from build123d import *

# Parameters (mm, degrees)
F0_W        = 0.9483136237
F0_H        = 3.3681727946
F0_W_2      = 28.0582979321
F0_H_2      = 55.2397826687
F0_W_3      = 6.7223012447
F0_H_3      = 9.4989053905
F0_H_4      = 10.2295875549
F0_W_4      = 6.8684406579
F0_W_5      = 7.014580071
F0_H_5      = 9.6450410783
F0_H_6      = 9.9373161793
F0_W_6      = 10.7689313591
F0_H_7      = 1.450072974
F0_W_7      = 10.0600272417
F1_DEPTH    = 2.54
F2_R        = 0.889
F3_DEPTH    = 1.778
F4_T4_DEPTH = 15.6041495789
F4_T9_DEPTH = 15.6041495789
F5_DEPTH    = 3.81
F6_DEPTH    = 3.302


# Not quite as in the source:
# - a fillet or chamfer that OpenCascade refuses, or shapes differently, is made with other operations: its cross-section is extruded or revolved along the edge and cut away or added


with BuildPart() as f1:
    # F0 (on Top) → F1 (new body)
    with BuildSketch(Plane.XY):
        with Locations((-55.3537514061, 60.8582701534)):
            Rectangle(F0_W, F0_H)
        Polygon((-69.7804093361, 57.7241107821), (-69.7804093361, 55.3859174252), (-41.8754070997, 55.3859174252), (-41.8754070997, 57.7241107821), (-44.8195673525, 57.7241107821), (-54.8795945942, 57.7241107821), (-55.8279082179, 57.7241107821), (-56.7762218416, 57.7241107821), (-67.5451532006, 57.7241107821), align=None)
        Polygon((-75.3612667322, 53.0477277935), (-69.7804093361, 53.0477277935), (-41.7221114039, 53.0477277935), (-35.9445475042, 53.0477277935), (-35.9445475042, 55.3859174252), (-41.8754070997, 55.3859174252), (-69.7804093361, 55.3859174252), (-75.3612667322, 55.3859174252), align=None)
        with Locations((-56.3020650297, 60.8582701534)):
            Rectangle(F0_W, F0_H)
        with Locations((-55.75126037, 25.4278364591)):
            Rectangle(F0_W_2, F0_H_2)
        with Locations((-62.9119724035, 14.8329045624)):
            Rectangle(F0_W_3, F0_H_3, mode=Mode.SUBTRACT)
        with Locations((-62.9119724035, 29.2273983359)):
            Rectangle(F0_W_3, F0_H_4, mode=Mode.SUBTRACT)
        with Locations((-48.2252072543, 14.8329045624)):
            Rectangle(F0_W_4, F0_H_3, mode=Mode.SUBTRACT)
        with Locations((-48.2252072543, 29.2273983359)):
            Rectangle(F0_W_4, F0_H_4, mode=Mode.SUBTRACT)
        with Locations((-63.0581118166, 44.571781531)):
            Rectangle(F0_W_5, F0_H_5, mode=Mode.SUBTRACT)
        with Locations((-48.2252072543, 44.4256439805)):
            Rectangle(F0_W_4, F0_H_6, mode=Mode.SUBTRACT)
        with Locations((-62.1606875211, 58.4491472691)):
            Rectangle(F0_W_6, F0_H_7)
        with Locations((-55.3537514061, 58.4491472691)):
            Rectangle(F0_W, F0_H_7)
        with Locations((-49.8495809734, 58.4491472691)):
            Rectangle(F0_W_7, F0_H_7)
        with Locations((-56.3020650297, 58.4491472691)):
            Rectangle(F0_W, F0_H_7)
    extrude(amount=F1_DEPTH)

    # F2
    f2_edges = [f1.edges().sort_by_distance(p)[0] for p in [
        (-54.879595, 60.85827, 2.54),
        (-56.776222, 60.85827, 2.54),
        (-55.827908, 62.542357, 2.54),
        (-56.776222, 62.542357, 1.27),
        (-54.879595, 62.542357, 1.27),
    ]]
    fillet(f2_edges, radius=F2_R)

    # F0 (on Top) → F3 (join)
    with BuildSketch(Plane.XY):
        with Locations((-63.0581118166, 44.571781531)):
            Rectangle(F0_W_5, F0_H_5)
        with Locations((-48.2252072543, 44.4256439805)):
            Rectangle(F0_W_4, F0_H_6)
        with Locations((-62.9119724035, 29.2273983359)):
            Rectangle(F0_W_3, F0_H_4)
        with Locations((-48.2252072543, 29.2273983359)):
            Rectangle(F0_W_4, F0_H_4)
        with Locations((-48.2252072543, 14.8329045624)):
            Rectangle(F0_W_4, F0_H_3)
        with Locations((-62.9119724035, 14.8329045624)):
            Rectangle(F0_W_3, F0_H_3)
    extrude(amount=F3_DEPTH)

    # F4: chamfer of 2.54 on 2 edges, made by hand


with BuildPart() as f4_tool2:
    # F4_s3 → F4_t4 (new body)
    with BuildSketch(Plane.XY.offset(-6.5320747894)):
        Polygon((-67.5451532006, 56.6341837561), (-65.0051532006, 59.1741837561), (-67.5451532006, 59.1741837561), align=None)
    extrude(amount=F4_T4_DEPTH)

    split(bisect_by=Plane.XZ.offset(-57.7241107821), keep=Keep.BOTTOM)


with BuildPart() as f1_1:
    add(f1.part)

    # F4_t1: cut F4_tool2
    add(f4_tool2.part, mode=Mode.SUBTRACT)


with BuildPart() as f4_tool7:
    # F4_s8 → F4_t9 (new body)
    with BuildSketch(Plane.XY.offset(-6.5320747894)):
        Polygon((-44.8195673525, 56.6341837561), (-47.3595673525, 59.1741837561), (-44.8195673525, 59.1741837561), align=None)
    extrude(amount=F4_T9_DEPTH)

    split(bisect_by=Plane.XZ.offset(-57.7241107821), keep=Keep.BOTTOM)


with BuildPart() as f1_2:
    add(f1_1.part)

    # F4_t6: cut F4_tool7
    add(f4_tool7.part, mode=Mode.SUBTRACT)

    # F0 (on Top) → F5 (join)
    with BuildSketch(Plane.XY):
        Polygon((-75.3612667322, 53.0477277935), (-69.7804093361, 53.0477277935), (-41.7221114039, 53.0477277935), (-35.9445475042, 53.0477277935), (-35.9445475042, 55.3859174252), (-41.8754070997, 55.3859174252), (-69.7804093361, 55.3859174252), (-75.3612667322, 55.3859174252), align=None)
    extrude(amount=F5_DEPTH)

    # F0 (on Top) → F6 (join)
    with BuildSketch(Plane.XY):
        Polygon((-69.7804093361, 57.7241107821), (-69.7804093361, 55.3859174252), (-41.8754070997, 55.3859174252), (-41.8754070997, 57.7241107821), (-44.8195673525, 57.7241107821), (-54.8795945942, 57.7241107821), (-55.8279082179, 57.7241107821), (-56.7762218416, 57.7241107821), (-67.5451532006, 57.7241107821), align=None)
    extrude(amount=F6_DEPTH)


solid = f1_2.part
Build history of the part. All positions in model axes, mm. A direction names the side the tool comes from. Round coordinates to 2 decimals unless told otherwise and drop trailing zeros. Write each loop counter-clockwise with the first axis right and the second up, starting at its lowest first coordinate (ties: lowest second). Pieces come first, ordered by that corner, then holes. Notation, with made-up numbers: (69.25, 36) -> (118.25, 36) arc R25 cw to (118.25, 52) -> close; hole circle Ø4 at (-35, 37). An arc over 180 degrees is marked (long way). Write item = value, one per line.
(1) Band-saw the part on B-B (y = 40.5). Give the cut face in (x, z), then the cut area to 3 significant figures.
Answer:
outline = (-69.78, 0) -> (-41.72, 0) -> (-41.72, 2.54) -> (-44.79, 2.54) -> (-44.79, 1.78) -> (-51.66, 1.78) -> (-51.66, 2.54) -> (-59.55, 2.54) -> (-59.55, 1.78) -> (-66.57, 1.78) -> (-66.57, 2.54) -> (-69.78, 2.54) -> close
area = 60.7 mm2
(2) Two-plate mould, pull along Y, no slides. Class faces 4 (the face through (-56, -2.192, 1)), 5 (the face through (-63, 45, 1.778)), 6 (the face through (-41.875, 57, 2)): pulls with the +Y half, pulls with the -Y half, needs draft (parallel to the pull), parting line crosses it, or undercut.
Answer:
face_4 = pulls with the -Y half
face_5 = undercut
face_6 = needs draft
(3) Band-saw the part on D-D (y = 31.5). Give the cut face in (x, z), then the cut area to 3 significant figures.
Answer:
outline = (-69.78, 0) -> (-41.72, 0) -> (-41.72, 2.54) -> (-44.79, 2.54) -> (-44.79, 1.78) -> (-51.66, 1.78) -> (-51.66, 2.54) -> (-59.55, 2.54) -> (-59.55, 1.78) -> (-66.27, 1.78) -> (-66.27, 2.54) -> (-69.78, 2.54) -> close
area = 60.9 mm2
(4) Tool access for faces 1 (the face through (-56.776, 60, 1)), 2 (the face through (-56, 26, 2.54)), 3 (the face through (-63, 15, 1.778)): list every direction of +Z, -Z, +X, -X, +Y, -Y with a clear straight run to the whole face (end or side of a thin tool).
Answer:
face_1 = +Z, -Z, -X, +Y
face_2 = +Z, +X, -X, -Y
face_3 = +Z
(5) Flat gauge pins, fed straight in: pin 1 (1.2 mm diameter, centred on y = 57, z = 2, fed in from -X); pin 2 (1 mm diameter, centred on x = -63, y = 38, fed in from +Z); pin 3 (0.6 mm diameter, centred on x = -62, z = 2, fed in from +Y). Where does each tip first touch, or does it go through?
Answer:
pin_1 = -69.78
pin_2 = 2.54
pin_3 = 59.17
(6) Band-saw the part on C-C (x = -61). Give the cut face in (y, z).
Answer:
outline = (-2.19, 0) -> (59.17, 0) -> (59.17, 2.54) -> (57.72, 2.54) -> (57.72, 3.3) -> (55.39, 3.3) -> (55.39, 3.81) -> (53.05, 3.81) -> (53.05, 2.54) -> (49.39, 2.54) -> (49.39, 1.78) -> (39.75, 1.78) -> (39.75, 2.54) -> (34.34, 2.54) -> (34.34, 1.78) -> (24.11, 1.78) -> (24.11, 2.54) -> (19.58, 2.54) -> (19.58, 1.78) -> (10.08, 1.78) -> (10.08, 2.54) -> (-2.19, 2.54) -> close
(7) Probe L1, parallel to Y at x = -57, z = 3.1; L2, parallel to Z at x = -42, y = 56; L3, parallel to Y at x = -42.5, z = 2.3. List the from-to ranges inside material, lowest first.
Answer:
L1 = 53.05 to 57.72
L2 = 0 to 3.3
L3 = -2.19 to 57.72
(8) Band-saw the part on A-A (x = -53.5). Give the cut face in (y, z).
Answer:
outline = (-2.19, 0) -> (59.17, 0) -> (59.17, 2.54) -> (57.72, 2.54) -> (57.72, 3.3) -> (55.39, 3.3) -> (55.39, 3.81) -> (53.05, 3.81) -> (53.05, 2.54) -> (-2.19, 2.54) -> close
